```python
from build123d import *

# Parameters (mm, degrees)
F0_R        = 2
F1_DEPTH    = 5
F2_T1_DEPTH = 30.7168298797
F2_T3_DEPTH = 16.2857086021
F3_SIZE     = 2
F4_SIZE     = 3
F5_SIZE     = 2


# Not quite as in the source:
# - a fillet or chamfer that OpenCascade refuses, or shapes differently, is made with other operations: its cross-section is extruded or revolved along the edge and cut away or added


with BuildPart() as f1:
    # F0 (on Front) → F1 (new body)
    with BuildSketch(Plane.XZ):
        Polygon((20, 0), (0, -20), (0, -90), (20, -90), (90, -20), (90, 0), align=None)
        with Locations((10, -80)):
            Circle(F0_R, mode=Mode.SUBTRACT)
        with BuildLine():
            Line((14, -31.908116908), (16.1091270347, -31.908116908))
            ThreePointArc((16.1091270347, -31.908116908), (17.6398607642, -32.2125987779), (18.9375541595, -33.0796897832))
            Line((18.9375541595, -33.0796897832), (38.0294372515, -52.1715728753))
            ThreePointArc((38.0294372515, -52.1715728753), (39.2010101268, -55), (38.0294372515, -57.8284271247))
            Line((38.0294372515, -57.8284271247), (23.8873016278, -71.9705627485))
            ThreePointArc((23.8873016278, -71.9705627485), (21.2333520525, -73.1383285101), (18.4877240643, -72.2063133962))
            Line((18.4877240643, -72.2063133962), (11.4288495613, -66.2832144042))
            ThreePointArc((11.4288495613, -66.2832144042), (10.3747688519, -64.9095096787), (10, -63.2190366317))
            Line((10, -63.2190366317), (10, -35.908116908))
            ThreePointArc((10, -35.908116908), (11.1715728753, -33.0796897832), (14, -31.908116908))
        make_face(mode=Mode.SUBTRACT)
        with Locations((47.9289321881, -47.9289321881)):
            Circle(F0_R, mode=Mode.SUBTRACT)
        with Locations((10, -24.1421356237)):
            Circle(F0_R, mode=Mode.SUBTRACT)
        with Locations((24.1421356237, -10)):
            Circle(F0_R, mode=Mode.SUBTRACT)
        with BuildLine():
            ThreePointArc((63.2190366317, -10), (64.9095096787, -10.3747688519), (66.2832144042, -11.4288495613))
            Line((66.2832144042, -11.4288495613), (72.2063133962, -18.4877240643))
            ThreePointArc((72.2063133962, -18.4877240643), (73.1383285101, -21.2333520525), (71.9705627485, -23.8873016278))
            Line((71.9705627485, -23.8873016278), (57.8284271247, -38.0294372515))
            ThreePointArc((57.8284271247, -38.0294372515), (55, -39.2010101268), (52.1715728753, -38.0294372515))
            Line((52.1715728753, -38.0294372515), (33.0796897832, -18.9375541595))
            ThreePointArc((33.0796897832, -18.9375541595), (32.2125987779, -17.6398607642), (31.908116908, -16.1091270347))
            Line((31.908116908, -16.1091270347), (31.908116908, -14))
            ThreePointArc((31.908116908, -14), (33.0796897832, -11.1715728753), (35.908116908, -10))
            Line((35.908116908, -10), (63.2190366317, -10))
        make_face(mode=Mode.SUBTRACT)
        with Locations((80, -10)):
            Circle(F0_R, mode=Mode.SUBTRACT)
    extrude(amount=F1_DEPTH)

    # F2: chamfer of 5 on 6 edges, made by hand

    # F2_s2 → F2_t1 (cut)
    with BuildSketch(Plane.XZ.offset(-12.8584149398)):
        Polygon((90, -5), (85, 0), (90, 0), align=None)
        Polygon((0, -85), (5, -90), (0, -90), align=None)
    extrude(amount=F2_T1_DEPTH, mode=Mode.SUBTRACT)

    # F2_s4 → F2_t3 (cut)
    with BuildSketch(Plane.XZ.offset(-5.6428543011)):
        Polygon((1.4644660941, -18.5355339059), (0, -22.0710678119), (0, -20), align=None)
        Polygon((18.5355339059, -1.4644660941), (22.0710678119, 0), (20, 0), align=None)
        Polygon((88.5355339059, -21.4644660941), (90, -17.9289321881), (90, -20), align=None)
        Polygon((17.9289321881, -90), (21.4644660941, -88.5355339059), (20, -90), align=None)
    extrude(amount=F2_T3_DEPTH, mode=Mode.SUBTRACT)

    # F3
    f3_edges = [f1.edges().sort_by_distance(p)[0] for p in [
        (0.732233, -5, -20.303301),
        (20.303301, -5, -0.732233),
        (10, -5, -10),
        (87.5, -5, -2.5),
        (89.267767, -5, -19.696699),
        (90, -5, -11.464466),
        (53.535534, -5, 0),
        (19.696699, -5, -89.267767),
        (2.5, -5, -87.5),
        (11.464466, -5, -90),
        (0, -5, -53.535534),
        (55, -5, -55),
    ]]
    chamfer(f3_edges, length=F3_SIZE)

    # F4
    f4_edges = [f1.edges().sort_by_distance(p)[0] for p in [
        (8, -5, -24.142136),
        (22.142136, -5, -10),
        (78, -5, -10),
        (45.928932, -5, -47.928932),
        (8, -5, -80),
    ]]
    chamfer(f4_edges, length=F4_SIZE)

    # F5
    f5_edges = [f1.edges().sort_by_distance(p)[0] for p in [
        (30.958369, -5, -64.899495),
        (21.233352, -5, -73.138329),
        (14.958287, -5, -69.244764),
        (10.374769, -5, -64.90951),
        (10, -5, -49.563577),
        (11.171573, -5, -33.07969),
        (17.639861, -5, -32.212599),
        (14, -2.5, -31.908117),
        (15.054564, -5, -31.908117),
        (28.483496, -5, -42.625631),
        (39.20101, -5, -55),
        (42.625631, -5, -28.483496),
        (33.07969, -5, -11.171573),
        (31.908117, -5, -15.054564),
        (49.563577, -5, -10),
        (32.212599, -5, -17.639861),
        (64.90951, -5, -10.374769),
        (69.244764, -5, -14.958287),
        (55, -5, -39.20101),
        (73.138329, -5, -21.233352),
        (64.899495, -5, -30.958369),
    ]]
    chamfer(f5_edges, length=F5_SIZE)


solid = f1.part
```
Part model, mm, in its own coordinate system. A direction names the side the tool comes from. Coordinates: 2 decimals unless noted, no trailing zeros. Write each loop counter-clockwise with the first axis right and the second up, starting at its lowest first coordinate (ties: lowest second). Pieces come first, ordered by that corner, then holes.
Item 1: Mould opens along X. For faces 4 (the face through (53.83, -3.99, -54.77)), 5 (the face through (11, -4, -89)), 6 (the face through (33.05, -1.48, -11.2)) say: released by +X, released by -X, zero draft, split by the parting line, or undercut.
Item 2: Slice it at C-C (y = -4.05). Count the separate pieces of the cut face and the enclosed holes in it, and give its area (3 significant figures).
Item 3: Slice it at B-B (x = 80). Write the cut outline in (y, z).
Item 4: Pin check, flat tips, straight feed: pin 1 (1 mm diameter, centred on x = 19, y = -4, fed in from -Z); pin 2 (5 mm diameter, centred on x = 80, z = -10, fed in from -Y); pin 3 (3.5 mm diameter, centred on x = 47.93, z = -47.93, fed in from -Y); pin 4 (2 mm diameter, centred on x = 55.5, y = -4, fed in from -Z). Stop position of each tip, or through.
Item 5: Which spindle directions (+Z, -Z, +X, -X, +Y, -Y) get a long thin tool onto all of the face, cutting with end or side? Do faces 1 (the face through (3.232, -3.986, -86.838)), 2 (the face through (55, -1.5, -39.2)), 3 (the face through (40, -3.8, -54.9)). Say none if no direction does.
Item 6: Probe line 1 (Z direction, x = 36, y = -2.2); line 2 (Z direction, x = 9.5, y = -4.2); line 3 (X direction, y = -3.95, z = -7.5). List the from-to ranges inside material, lowest first.
Item 7: Slice it at A-A (z = -80). Write the cut outline in (x, y), and give its area (3 significant figures).
Results found:
1. face 4: released by +X
1. face 5: zero draft
1. face 6: undercut
2. separate pieces: 1
2. enclosed holes: 7
2. area: 3,020 mm2
3. outline: (-5, -27.17) - (-3, -30) - (0, -30) - (0, -12) - (-2, -12) - (-5, -15) - close; (-5, -5) - (-2, -8) - (0, -8) - (0, 0) - (-3, 0) - (-5, -2) - close
4. pin 1: stops at z = -89.05
4. pin 2: stops at y = -2.5
4. pin 3: passes through
4. pin 4: stops at z = -54.82
5. face 1: -Z, -X, -Y
5. face 2: +Y, -Y
5. face 3: -Y
6. line 1: z = -74 to -59.86, -50.14 to -21.86, -10 to 0
6. line 2: z = -88.8 to -84.17, -75.83 to -65.82, -33.3 to -28.31, -19.97 to -12.2
6. line 3: x = 13.84 to 21.08, 27.2 to 76.94, 83.06 to 89.05
7. outline: (0, -3) - (2, -5) - (5, -5) - (8, -2) - (8, 0) - (0, 0) - close; (12, -2) - (15, -5) - (27.17, -5) - (30, -3) - (30, 0) - (12, 0) - close
7. area: 116 mm2
